Can you work these out from the model? Positions are in its coordinate system, mm. A direction names the side the tool comes from. Give positions to 0.01 mm unless a question says otherwise; leave off trailing zeros. Order: outer loops, then holes, each group sorted by start corner. A loop starts at its lowest first (then second) coordinate and runs counter-clockwise, first axis right, second up. Notation, with made-up numbers: (-8, -20) - (8, -20) arc R27 ccw to (8, 15) - close; hole circle Ø6 at (8.25, 3.5). An arc over 180 degrees is marked (long way). Return JSON: item names as keys, results as strings.
```python
from build123d import *

# Parameters (mm, degrees)
SKETCH_1_W          = 200
SKETCH_1_H          = 100
EXTRUDE_1_DEPTH     = 90
SKETCH_2_W          = 20
SKETCH_2_H          = 20
CUT_EXTRUDE_1_DEPTH = 200
FILLET_1_R          = 10
SHELL_1_T           = -3
FILLET_2_R          = 3
SKETCH_3_R          = 3
CUT_EXTRUDE_2_DEPTH = 3


with BuildPart() as part:
    # 草圖1 → 填料-伸長1 (new body)
    with BuildSketch(Plane(origin=(0, 0, 0), x_dir=(1, 0, 0), z_dir=(0, 1, 0))):
        Rectangle(SKETCH_1_W, SKETCH_1_H)
    extrude(amount=EXTRUDE_1_DEPTH)

    # 草圖2 → 除料-伸長1 (cut)
    with BuildSketch(Plane(origin=(100, 0, 0), x_dir=(0, 0, -1), z_dir=(1, 0, 0))):
        with Locations((40, 10)):
            Rectangle(SKETCH_2_W, SKETCH_2_H)
    extrude(amount=-CUT_EXTRUDE_1_DEPTH, mode=Mode.SUBTRACT)

    # 圓角1
    fillet_1_edges = [part.edges().sort_by_distance(p)[0] for p in [
        (-100, 0, 10),
        (100, 0, 10),
    ]]
    fillet(fillet_1_edges, radius=FILLET_1_R)

    # 薄殼1
    shell_1_openings = [part.faces().sort_by_distance(p)[0] for p in [
        (0, 90, 0),
    ]]
    offset(amount=SHELL_1_T, openings=shell_1_openings, kind=Kind.INTERSECTION)

    # 圓角2
    fillet_2_edges = [part.edges().sort_by_distance(p)[0] for p in [
        (0, 0, 50),
        (97.071067812, 2.928932188, 50),
        (-97.071067812, 2.928932188, 50),
        (97, 50, 47),
        (97, 56.5, -47),
        (-97, 56.5, -47),
        (-97, 50, 47),
        (-94.949747468, 5.050252532, 47),
        (0, 3, 47),
        (94.949747468, 5.050252532, 47),
        (100, 50, 50),
        (-100, 50, 50),
        (-100, 55, -50),
        (100, 55, -50),
    ]]
    fillet(fillet_2_edges, radius=FILLET_2_R)

    # 草圖3 → 除料-伸長2 (cut)
    with BuildSketch(Plane(origin=(0, 23, 0), x_dir=(1, 0, 0), z_dir=(0, 1, 0))):
        with Locations(Location((-35, 37, 0), (0, 0, 270))):
            Circle(SKETCH_3_R)
        with Locations(Location((35, 37, 0), (0, 0, 270))):
            Circle(SKETCH_3_R)
    extrude(amount=-CUT_EXTRUDE_2_DEPTH, mode=Mode.SUBTRACT)


solid = part.part
```
1. For pin 1 Ø10 at (x, y) = (-46, 12) entering from -Z; pin 2 Ø8 at (x, z) = (-35, -37) entering from +Y; pin 3 Ø8 at (x, z) = (35, -37) entering from -Y; pin 4 Ø22 at (x, z) = (3.5, -37) entering from -Y, each with a flat end and sliding along its axis, tell me the tip position at first contact or that it passes through.
Checks:
{"pin 1": "z = -30", "pin 2": "y = 23", "pin 3": "y = 20", "pin 4": "y = 0"}
2. On a 3-axis mill with a long thin cutter (end or side, diameter ignored), from which of +Z, -Z, +X, -X, +Y, -Y can I reach the whole of each face in a straight line? I mean faces 1 (the face through (1, 10, -30)), 2 (the face through (-1, 47, 47)), 3 (the face through (-1, 0, 8)). Say none if no direction works.
Checks:
{"face 1": "-Z, +X, -X, -Y", "face 2": "+Y", "face 3": "+Z, -Z, +X, -X, -Y"}
3. Suppose I cut it at D-D (x = 74). List the corners of the cut face in (y, z) for me, plus the area to 3 significant figures.
Checks:
{"outline": "(0, -30) - (20, -30) - (20, -50) - (90, -50) - (90, -47) - (23, -47) - (23, -27) - (3, -27) - (3, 44) arc R3 cw to (6, 47) - (90, 47) - (90, 50) - (3, 50) arc R3 ccw to (0, 47) - close", "area": "822 mm^2"}
4. Suppose I cut it at B-B (z = -36.5). List the corners of the cut face in (x, y) for me.
Checks:
{"outline": "(-100, 20) - (-37.96, 20) - (-37.96, 23) - (-97, 23) - (-97, 90) - (-100, 90) - close; (-32.04, 20) - (32.04, 20) - (32.04, 23) - (-32.04, 23) - close; (37.96, 20) - (100, 20) - (100, 90) - (97, 90) - (97, 23) - (37.96, 23) - close"}
5. Suppose I cut it at C-C (y = 43.5). List the corners of the cut face in (x, z) for me, plus the area to 3 significant figures.
Checks:
{"outline": "(-100, -47) arc R3 ccw to (-97, -50) - (97, -50) arc R3 ccw to (100, -47) - (100, 47) arc R3 ccw to (97, 50) - (-97, 50) arc R3 ccw to (-100, 47) - close; hole (-97, -44) arc R3 ccw to (-94, -47) - (94, -47) arc R3 ccw to (97, -44) - (97, 44) arc R3 ccw to (94, 47) - (-94, 47) arc R3 ccw to (-97, 44) - close", "area": "1,760 mm^2"}
6. Thinking about a two-plate mould opening in Z: for faces 4 (the face through (1, 13, -27)), 5 (the face through (-1, 55, -50)), 6 (the face through (-100, 49, 1)), which applies, +Z half, -Z half, draft (parallel to the pull), parting line (faces both ways), or undercut?
Checks:
{"face 4": "undercut", "face 5": "-Z half", "face 6": "draft"}
7. If I drill on L1, parallel to X at y = 22, z = -37; L2, parallel to Z at x = -61, y = 66.5; L3, parallel to X at y = 55.5, z = 30, over which ranges is the centre line in solid material (lowest first)? Write a range as [from, to].
Checks:
{"L1": "[-100, -38], [-32, 32], [38, 100]", "L2": "[-50, -47], [47, 50]", "L3": "[-100, -97], [97, 100]"}
8. Suppose I cut it at A-A (x = 35). List the corners of the cut face in (y, z) for me.
Checks:
{"outline": "(0, -30) - (20, -30) - (20, -34) - (23, -34) - (23, -27) - (3, -27) - (3, 44) arc R3 cw to (6, 47) - (90, 47) - (90, 50) - (3, 50) arc R3 ccw to (0, 47) - close; (20, -50) - (90, -50) - (90, -47) - (23, -47) - (23, -40) - (20, -40) - close"}
